```python
from build123d import *

# Parameters (mm, degrees)
F0_W     = 80.35636
F0_H     = 77.816363
F1_DEPTH = 12.7
F2_W     = 9.929092
F2_H     = 9.005454
F3_DEPTH = 76.2
F4_W     = 10.160005
F4_H     = 9.005454
F5_DEPTH = 76.2
F6_W     = 7.158185
F6_H     = 8.543637
F7_DEPTH = 76.2
F8_W     = 8.081818
F8_H     = 9.698183
F9_DEPTH = 76.2


with BuildPart() as f1:
    # F0 (on Front) → F1 (new body)
    with BuildSketch(Plane.XZ):
        with Locations((1.965884, -2.309089)):
            Rectangle(F0_W, F0_H)
    extrude(amount=F1_DEPTH)

    # F2 (on Front) → F3 (join)
    with BuildSketch(Plane.XZ):
        with Locations((-30.364546, 27.709091)):
            Rectangle(F2_W, F2_H)
    extrude(amount=F3_DEPTH)

    # F4 (on Front) → F5 (join)
    with BuildSketch(Plane.XZ):
        with Locations((28.632728, 26.323637)):
            Rectangle(F4_W, F4_H)
    extrude(amount=F5_DEPTH)

    # F6 (on Front) → F7 (join)
    with BuildSketch(Plane.XZ):
        with Locations((-30.133637, -32.096365)):
            Rectangle(F6_W, F6_H)
    extrude(amount=F7_DEPTH)

    # F8 (on Front) → F9 (join)
    with BuildSketch(Plane.XZ):
        with Locations((26.670001, -31.28818)):
            Rectangle(F8_W, F8_H)
    extrude(amount=F9_DEPTH)


solid = f1.part
```
Verification items for the finished model (mm, model axes). A direction names the side the tool comes from. Round coordinates to 2 decimals unless told otherwise and drop trailing zeros. Write each loop counter-clockwise with the first axis right and the second up, starting at its lowest first coordinate (ties: lowest second). Pieces come first, ordered by that corner, then holes.
1. Section check D-D on z = -4.5. Enter the section's corners in (x, y), plus the area to 3 significant figures.
2. Scan lines: L1, parallel to X at y = -47, z = 24; L2, parallel to X at y = -13.5, z = -34; L3, parallel to Z at x = 29.5, y = -67.5. Record each from-to range of solid material in increasing order.
3. Section check A-A on y = -29. Enter the section's corners in (x, z), plus the area to 3 significant figures.
4. Section check B-B on z = 24.5. Enter the section's corners in (x, y), plus the area to 3 significant figures.
5. Section check C-C on x = -1. Enter the section's corners in (y, z).
6. Draft check along X on faces 1 (the flat face through (30.711, -44, -31)), 2 (the flat face through (-33.713, -44, -32)), 3 (the flat face through (22.629, -44, -31)), 4 (the flat face through (-30, -44, -36.368)). Enter one of: +X half, -X half, draft (parallel to the pull), parting line (faces both ways), or undercut.
7. Gauge pin test, flat ends, axial feed: P1, Ø2.5, axis at y = -41.5, z = 28, coming from the -X side; P2, Ø7, axis at y = -56.5, z = -30.5, coming from the +X side; P3, Ø9, axis at x = 25.5, y = -35.5, coming from the +Z side. Record the tip position at first contact, or that the pin passes through.
8. Access from +Z, -Z, +X, -X, +Y, -Y to the whole of each face (thin tool, end or side, straight path). Record for faces 5 (the flat face through (-30, -44, 32.212)), 6 (the flat face through (-30, -44, 23.206)), 7 (the flat face through (29, -44, 30.826)).
Answer:
1. outline: (-38.21, -12.7) - (42.14, -12.7) - (42.14, 0) - (-38.21, 0) - close
1. area: 1,020 mm2
2. L1: x = -35.33 to -25.4, 23.55 to 33.71
2. L2: x = -33.71 to -26.55, 22.63 to 30.71
2. L3: z = -36.14 to -26.44, 21.82 to 30.83
3. outline: (-35.33, 23.21) - (-25.4, 23.21) - (-25.4, 32.21) - (-35.33, 32.21) - close; (-33.71, -36.37) - (-26.55, -36.37) - (-26.55, -27.82) - (-33.71, -27.82) - close; (22.63, -36.14) - (30.71, -36.14) - (30.71, -26.44) - (22.63, -26.44) - close; (23.55, 21.82) - (33.71, 21.82) - (33.71, 30.83) - (23.55, 30.83) - close
3. area: 320 mm2
4. outline: (-38.21, -12.7) - (-35.33, -12.7) - (-35.33, -76.2) - (-25.4, -76.2) - (-25.4, -12.7) - (23.55, -12.7) - (23.55, -76.2) - (33.71, -76.2) - (33.71, -12.7) - (42.14, -12.7) - (42.14, 0) - (-38.21, 0) - close
4. area: 2,300 mm2
5. outline: (-12.7, -41.22) - (0, -41.22) - (0, 36.6) - (-12.7, 36.6) - close
6. face 1: +X half
6. face 2: -X half
6. face 3: undercut
6. face 4: draft
7. P1: stops at x = -35.33
7. P2: stops at x = 30.71
7. P3: stops at z = 30.83
8. face 5: +Z, +X, -X, -Y
8. face 6: -X, -Y
8. face 7: +Z, +X, -Y
